from build123d import *

# Parameters (mm, degrees)
EXTRUSION1_DEPTH        = 3
ESQUISSE2_R             = 1.5
ENL_V_MAT_EXTRU_1_DEPTH = 16
ESQUISSE3_R             = 5
ENL_V_MAT_EXTRU_2_DEPTH = 16
ESQUISSE4_R             = 5
ENL_V_MAT_EXTRU_3_DEPTH = 16
ESQUISSE5_R             = 1.5
ENL_V_MAT_EXTRU_4_DEPTH = 25.792218749
ESQUISSE8_R             = 3
ENL_V_MAT_EXTRU_5_DEPTH = 8
ESQUISSE9_R             = 1.5
ENL_V_MAT_EXTRU_6_DEPTH = 10
ESQUISSE11_W            = 10
ESQUISSE11_H            = 5
ENL_V_MAT_EXTRU_9_DEPTH = 0.0001


with BuildPart() as part:
    # Esquisse1 → Extrusion1 (new body)
    with BuildSketch(Plane.XY):
        Polygon((0, 0), (-120, 0), (-120, -150), (-70, -200), (-50, -200), (0, -150), align=None)
    extrude(amount=EXTRUSION1_DEPTH)

    # Esquisse2 → Enlèv. mat.-Extru.1 (cut)
    with BuildSketch(Plane.XY):
        with Locations(Location((-69.5, -81.5, 0), (0, 0, 180))):
            Circle(ESQUISSE2_R)
        with Locations(Location((-41.5, -81.5, 0), (0, 0, 180))):
            Circle(ESQUISSE2_R)
        with Locations(Location((-74, -135, 0), (0, 0, 180))):
            Circle(ESQUISSE2_R)
        with Locations(Location((-24, -135, 0), (0, 0, 180))):
            Circle(ESQUISSE2_R)
    extrude(amount=ENL_V_MAT_EXTRU_1_DEPTH, mode=Mode.SUBTRACT)

    # Esquisse3 → Enlèv. mat.-Extru.2 (cut)
    with BuildSketch(Plane(origin=(0, 0, 0), x_dir=(-1, 0, 0), z_dir=(0, 0, -1))):
        with Locations((50, -60)):
            Circle(ESQUISSE3_R)
    extrude(amount=-ENL_V_MAT_EXTRU_2_DEPTH, mode=Mode.SUBTRACT)

    # Esquisse4 → Enlèv. mat.-Extru.3 (cut)
    with BuildSketch(Plane(origin=(0, 0, 0), x_dir=(-1, 0, 0), z_dir=(0, 0, -1))):
        with Locations((60, -10)):
            Circle(ESQUISSE4_R)
        with Locations((10, -85)):
            Circle(ESQUISSE4_R)
        with Locations((110, -85)):
            Circle(ESQUISSE4_R)
    extrude(amount=-ENL_V_MAT_EXTRU_3_DEPTH, mode=Mode.SUBTRACT)

    # Esquisse5 → Enlèv. mat.-Extru.4 (cut)
    with BuildSketch(Plane.XY):
        with Locations(Location((-97, -40, 0), (0, 0, 180))):
            Circle(ESQUISSE5_R)
        with Locations(Location((-63, -40, 0), (0, 0, 180))):
            Circle(ESQUISSE5_R)
        with Locations(Location((-63, -64, 0), (0, 0, 180))):
            Circle(ESQUISSE5_R)
        with Locations(Location((-97, -64, 0), (0, 0, 180))):
            Circle(ESQUISSE5_R)
    extrude(amount=ENL_V_MAT_EXTRU_4_DEPTH, mode=Mode.SUBTRACT)

    # Esquisse8 → Enlèv. mat.-Extru.5 (cut)
    with BuildSketch(Plane(origin=(0, 0, 0), x_dir=(-1, 0, 0), z_dir=(0, 0, -1))):
        with Locations((52.5, -23)):
            Circle(ESQUISSE8_R)
        with Locations((42.5, -23)):
            Circle(ESQUISSE8_R)
        with Locations((67.5, -23)):
            Circle(ESQUISSE8_R)
        with Locations((77.5, -23)):
            Circle(ESQUISSE8_R)
    extrude(amount=-ENL_V_MAT_EXTRU_5_DEPTH, mode=Mode.SUBTRACT)

    # Esquisse9 → Enlèv. mat.-Extru.6 (cut)
    with BuildSketch(Plane(origin=(0, 0, 0), x_dir=(-1, 0, 0), z_dir=(0, 0, -1))):
        with Locations((60, -152)):
            Circle(ESQUISSE9_R)
        with Locations((60, -197)):
            Circle(ESQUISSE9_R)
    extrude(amount=-ENL_V_MAT_EXTRU_6_DEPTH, mode=Mode.SUBTRACT)

    # Esquisse11 → Enlèv. mat.-Extru.9 (cut)
    with BuildSketch(Plane.XY.offset(3)):
        with Locations((-115, -23)):
            Rectangle(ESQUISSE11_W, ESQUISSE11_H)
        with Locations((-5, -23)):
            Rectangle(ESQUISSE11_W, ESQUISSE11_H)
    extrude(amount=-ENL_V_MAT_EXTRU_9_DEPTH, mode=Mode.SUBTRACT)


solid = part.part
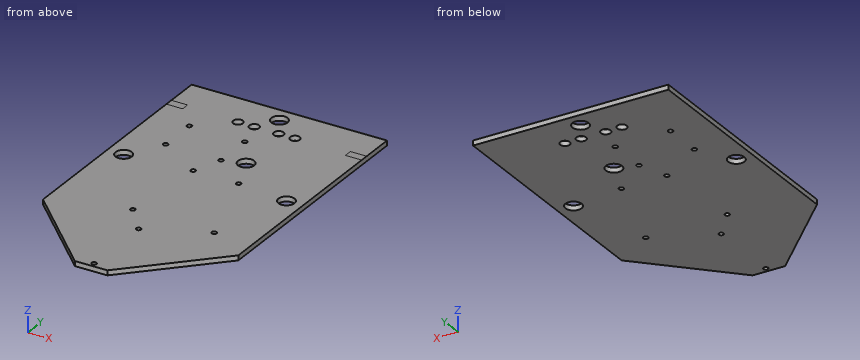
Here's how the part is built. I have some questions about the finished solid (model axes, mm). Give positions to 0.01 mm unless a question says otherwise; leave off trailing zeros. Loops run counter-clockwise (first coordinate to the right, second up) from the corner with the lowest first, then second, coordinate; pieces in that order, holes last. Notation, with made-up numbers: (8, -23) -> (64, -23) arc R17 ccw to (64, -12) -> close; hole circle Ø11 at (-12.75, 9.5). An arc over 180 degrees is marked (long way). One line per item, written item: value.
Q1. I'm going to push flat-ended pins straight in: pin 1 Ø3.5 at (x, y) = (-52.5, -23) entering from -Z (1 decimal); pin 2 Ø13 at (x, y) = (-60, -10) entering from -Z. Where does each tip first touch, or does it pass through?
Answers follow:
pin 1: through
pin 2: z = 0
Q2. If I drill on line 1 along X through (y, z) = (-40, 1.7); line 2 along X through (y, z) = (-135, 0.9); line 3 along Y through (x, z) = (-60, 1.1), over which ranges is the centre line in solid material (lowest first)?
Answers follow:
line 1: -120 to -98.5, -95.5 to -64.5, -61.5 to 0
line 2: -120 to -75.5, -72.5 to -25.5, -22.5 to 0
line 3: -200 to -198.5, -195.5 to -153.5, -150.5 to -15, -5 to 0
Q3. Suppose I cut it at D-D on y = -60. Please give me the cut outline in (x, z), then the cut area to 3 significant figures.
Answers follow:
outline: (-120, 0) -> (-55, 0) -> (-55, 3) -> (-120, 3) -> close; (-45, 0) -> (0, 0) -> (0, 3) -> (-45, 3) -> close
area: 330 mm^2
Q4. Suppose I cut it at C-C on x = -53. Please give me the cut outline in (y, z).
Answers follow:
outline: (-200, 0) -> (-64, 0) -> (-64, 3) -> (-200, 3) -> close; (-56, 0) -> (-25.96, 0) -> (-25.96, 3) -> (-56, 3) -> close; (-20.04, 0) -> (0, 0) -> (0, 3) -> (-20.04, 3) -> close
Q5. Suppose I cut it at A-A on y = -23. State how many separate pieces and enclosed holes the cut face has, then the cut area to 3 significant figures.
Answers follow:
separate pieces: 5
enclosed holes: 0
area: 288 mm^2
